Verification items for the finished model (mm, model axes). Face numbers are marked on the shaded views. A direction names the side the tool comes from. Give positions to 0.01 mm unless a question says otherwise; leave off trailing zeros. Loops run counter-clockwise (first coordinate to the right, second up) from the corner with the lowest first, then second, coordinate; pieces in that order, holes last. Notation, with made-up numbers: (-24, 89) -> (16, 89) arc R20 ccw to (16, 120) -> close; hole circle Ø7 at (71.25, -33). An arc over 180 degrees is marked (long way). Answer in a Markdown table with one row per item. Add a question column.
Q1. Material ranges on probe 1 along Z at (x, y) = (21.5, 0); probe 2 along Z at (x, y) = (18, 0); probe 3 along X at (y, z) = (0, 222.5), recorded low to high.
Q2. Section check B-B on z = 38. Enter the section's corners in (x, y).
Q3. Set-up check for the marked faces 1 and 2: record each of +Z, -Z, +X, -X, +Y, -Y from which the full face is reachable in a straight line by a thin tool's end or side.
Q4. Gauge pin test, flat ends, axial feed: P1, Ø3, axis at x = 10, y = 23.5, coming from the -Z side; P2, Ø3, axis at y = 17, z = 67, coming from the -X side; P3, Ø3, axis at y = 9, z = 125.5, coming from the +X side. Record the tip position at first contact, or that the pin passes through.
Q5. Section check A-A on z = 192. Enter the section's corners in (x, y).
Solid Edge part; units mm, degrees
sketch "Sketch1" plane through (0, 0, 0) normal (0, -1, 0) x (1, 0, 0)
  line L0 (32.5, 157) -> (32.5, 227)
  line L1 (32.5, 227) -> (11, 227)
  line L2 (11, 227) -> (11, 240)
  line L3 (11, 240) -> (0, 240)
  line L4 (0, 0) -> (0, 240)
  line L5 (0, 0) -> (19, 0)
  line L6 (19, 0) -> (19, 157)
  line L7 (19, 157) -> (32.5, 157)
revolve "RevolvedProtrusion1" add sketch "Sketch1" angle 360 about axis through (0, 0, 0) along (0, 0, 1)
chamfer "Chamfer1" distance 10 angle 45 1 edges at (-32.5, 0, 157)
chamfer "Chamfer_2" distance 10 angle 45 1 edges at (-32.5, 0, 227)
cosmetic_thread "Thread_1" thread depth 154
chamfer "Chamfer_4" distance 1 angle 45 1 edges at (-19, 0, 0)
hole "DRILL_Hole" at (0, 0, 240) direction (0, 0, -1) diameter 10.106 depth 35 tip angle 118 thread major 12 thread length 2
sketch "Sketch2" plane through (0, 0, 0) normal (0, -1, 0) x (1, 0, 0)
  circle A0 centre (0, 192) radius 6
extrude "Cutout1" cut sketch "Sketch2" along normal through all and the other way through all
sketch "Sketch3" plane through (0, 0, 0) normal (1, 0, 0) x (0, 1, 0)
  circle A0 centre (0, 192) radius 6
extrude "Cutout2" cut sketch "Sketch3" along normal through all and the other way through all
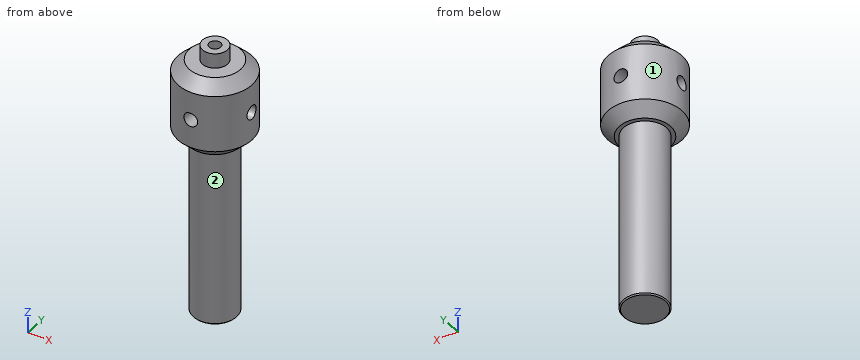
Taken from the geometry:
| question | item | result |
|---|---|---|
| 1 | probe 1 | z = 157 to 186, 198 to 227 |
| 1 | probe 2 | z = 0 to 186, 198 to 227 |
| 1 | probe 3 | x = -27 to -5.05, 5.05 to 27 |
| 2 | outline | circle Ø38 at (0, 0) |
| 3 | face 1 | +Z, -Z |
| 3 | face 2 | -Z |
| 4 | P1 | stops at z = 158.54 |
| 4 | P2 | stops at x = -10.99 |
| 4 | P3 | stops at x = 17.46 |
| 5 | outline | (-31.94, -6) arc R32.5 ccw to (-6, -31.94) -> (-6, -6) -> close; (-31.94, 6) -> (-6, 6) -> (-6, 31.94) arc R32.5 ccw to start; (6, -31.94) arc R32.5 ccw to (31.94, -6) -> (6, -6) -> close; (6, 6) -> (31.94, 6) arc R32.5 ccw to (6, 31.94) -> close |
